Check sheet for the modelled part. Datum: model origin and axes. Units: mm. A direction names the side the tool comes from. Round coordinates to 2 decimals unless told otherwise and drop trailing zeros. Write each loop counter-clockwise with the first axis right and the second up, starting at its lowest first coordinate (ties: lowest second). Pieces come first, ordered by that corner, then holes.
Item 1: Set-up check for faces 4 (the flat face through (-18, 17, 5)), 5 (the flat face through (-18, -16, 5)), 6 (the cylindrical face through (-1.301, 19.143, 4.93)): record each of +Z, -Z, +X, -X, +Y, -Y from which the full face is reachable in a straight line by a thin tool's end or side.
Item 2: Section check A-A, the plane y = 0. Record the cut outline in (x, z).
Item 3: Material ranges on line 1 along Y through (x, z) = (0, 2.5); line 2 along Z through (x, y) = (-60, 4.25); line 3 along Y through (x, z) = (-65, 40), recorded low to high.
Item 4: Section check D-D, the plane x = 0. Record the cut outline in (y, z), plus the area to 4 significant figures.
Item 5: Section check C-C, the plane z = 22. Record the cut outline in (x, y), plus the area to 3 significant figures.
Item 6: Depth check by flat-ended pin: pin 1 (1.5 mm diameter, centred on x = -50, z = 26.5, fed in from -Y); pin 2 (4 mm diameter, centred on y = 5.5, z = 9.5, fed in from +X); pin 3 (3 mm diameter, centred on y = -17.5, z = 3.5, fed in from -X). Enter the tip coordinate at first touch or a pass-through.
Item 7: Section check B-B, the plane x = -63. Record the cut outline in (y, z).
Item 8: Release check for a two-part mould opening along Y. For faces 1 (the cylindrical face through (30.63, 23.09, 4.93)), 2 (the cylindrical face through (44, 0, 5)), 3 (the flat face through (15, 10, 10)) record: pulls with the +Y half, pulls with the -Y half, needs draft (parallel to the pull), parting line crosses it, or undercut.
from build123d import *

# Parameters (mm, degrees)
F0_R     = 6
F1_DEPTH = 10
F2_R     = 10
F3_DEPTH = 8
F4_DEPTH = 8


with BuildPart() as f1:
    # F0 (on Top) → F1 (new body)
    with BuildSketch(Plane.XY):
        with BuildLine():
            ThreePointArc((50.720724, -17.985565), (68, 0), (50.720724, 17.985565))
            ThreePointArc((50.720724, 17.985565), (30.362055, 23.224109), (13.956018, 36.367918))
            ThreePointArc((13.956018, 36.367918), (-6.032896, 41.958896), (-18, 25))
            Line((-18, 25), (-18, -25))
            ThreePointArc((-18, -25), (-6.032896, -41.958896), (13.956018, -36.367918))
            ThreePointArc((13.956018, -36.367918), (30.362055, -23.224109), (50.720724, -17.985565))
        make_face()
        with Locations((0, -25)):
            Circle(F0_R, mode=Mode.SUBTRACT)
        with Locations((0, 25)):
            Circle(F0_R, mode=Mode.SUBTRACT)
        with Locations((50, 0)):
            Circle(F0_R, mode=Mode.SUBTRACT)
    extrude(amount=F1_DEPTH)

    # F2 (on Front) → F3 (join)
    with BuildSketch(Plane.XZ):
        with BuildLine():
            ThreePointArc((-45.928789, 38.911565), (-80.688818, 29.481496), (-60, 0))
            Line((-60, 0), (34.021274, 0))
            Line((34.021274, 0), (34.021274, 10))
            ThreePointArc((34.021274, 10), (-8.487228, 17.449895), (-45.928789, 38.911565))
        make_face()
        with Locations((-60, 22)):
            Circle(F2_R, mode=Mode.SUBTRACT)
    extrude(amount=F3_DEPTH)

    # F2 (on Front) → F4 (join)
    with BuildSketch(Plane.XZ):
        with BuildLine():
            ThreePointArc((-45.928789, 38.911565), (-80.688818, 29.481496), (-60, 0))
            Line((-60, 0), (34.021274, 0))
            Line((34.021274, 0), (34.021274, 10))
            ThreePointArc((34.021274, 10), (-8.487228, 17.449895), (-45.928789, 38.911565))
        make_face()
        with Locations((-60, 22)):
            Circle(F2_R, mode=Mode.SUBTRACT)
    extrude(amount=-F4_DEPTH)


solid = f1.part
Values found:
1. face 4: +Z, -Z, -X, +Y
1. face 5: +Z, -Z, -X, -Y
1. face 6: +Z, -Z
2. outline: (-60, 0) - (44, 0) - (44, 10) - (34.02, 10) arc R125 cw to (-45.93, 38.91) arc R22 ccw (long way) to start; (56, 0) - (68, 0) - (68, 10) - (56, 10) - close; hole circle Ø20 at (-60, 22)
3. line 1: y = -43 to -31, -19 to 19, 31 to 43
3. line 2: z = 0 to 12, 32 to 44
3. line 3: y = -8 to 8
4. outline: (-43, 0) - (-31, 0) - (-31, 10) - (-43, 10) - close; (-19, 0) - (19, 0) - (19, 10) - (8, 10) - (8, 14.72) - (-8, 14.72) - (-8, 10) - (-19, 10) - close; (31, 0) - (43, 0) - (43, 10) - (31, 10) - close
4. area: 695.5 mm2
5. outline: (-82, -8) - (-70, -8) - (-70, 8) - (-82, 8) - close; (-50, -8) - (-19.42, -8) - (-19.42, 8) - (-50, 8) - close
5. area: 681 mm2
6. pin 1: stops at y = -8
6. pin 2: stops at x = 67.66
6. pin 3: stops at x = -18
7. outline: (-8, 0.21) - (8, 0.21) - (8, 12.46) - (-8, 12.46) - close; (-8, 31.54) - (8, 31.54) - (8, 43.79) - (-8, 43.79) - close
8. face 1: pulls with the +Y half
8. face 2: undercut
8. face 3: needs draft
